Model file for the job. Use its own axes, mm. A direction names the side the tool comes from. Coordinates: 2 decimals unless noted, no trailing zeros. Order: outer loops, then holes, each group sorted by start corner. A loop starts at its lowest first (then second) coordinate and runs counter-clockwise, first axis right, second up. Notation, with made-up numbers: (5.5, 3) -> (30.5, 3) arc R27 cw to (30.5, 27) -> close; hole circle Ø1 at (87.5, 15). An arc over 180 degrees is marked (long way). Return JSON: item names as keys, results as strings. Group by question number.
1) Cut at B-B (z = 5). Write the cut outline in (x, y).
2) Flat gauge pins, fed straight in: pin 1 (5.5 mm diameter, centred on x = -1, y = 4, fed in from +Z); pin 2 (6 mm diameter, centred on x = -8, y = 9.5, fed in from +Z); pin 3 (5.5 mm diameter, centred on x = 14, z = 15, fed in from +Y); pin 4 (2 mm diameter, centred on x = -16, y = 5.5, fed in from +Z). Where does each tip first touch, or does it go through?
3) Cut at A-A (y = 5). Write the cut outline in (x, z).
4) Probe line 1 (Z direction, x = -14, y = 3.5); line 2 (Z direction, x = -12, y = 13.75); line 3 (X direction, y = 3.25, z = 57.5). List the from-to ranges inside material, lowest first.
5) Which spindle directions (+Z, -Z, +X, -X, +Y, -Y) get a long thin tool onto all of the face, cutting with end or side? Do faces 4 (the flat face through (0, 10, 11)), 5 (the cylindrical face through (10.925, 14.014, 126.686)), 6 (the flat face through (0.2, 9.3, 20)). Say none if no direction does.
6) Pull direction X, two halves, no side cores. Call faces 1 (the flat face through (-0.2, 9.3, 0)), 2 (the flat face through (-15.5, 6, 71)), 3 (the flat face through (-17.5, 8, 66)): +X half, -X half, draft (parallel to the pull), parting line (faces both ways), or undercut.
7) Cut at C-C (z = 76). Write the cut outline in (x, y).
8) Cut at D-D (x = -0.5). Write the cut outline in (y, z).
Autodesk Fusion 360 part; units mm, degrees
sketch "スケッチ1" plane through (0, 0, 0) normal (0, 0, 1) x (1, 0, 0)
  line L0 (-17.5, 15) -> (17.5, 15)
  line L1 (17.5, 15) -> (17.5, 0)
  line L2 (17.5, 0) -> (-17.5, 0)
  line L3 (-17.5, 0) -> (-17.5, 15)
  dimension "d1" = 35
  dimension "d2" = 15
extrude "押し出し1" add sketch "スケッチ1" along normal blind 120
sketch "スケッチ2" plane through (0, 0, 0) normal (0, 0, -1) x (1, 0, 0)
  line L0 (17.5, 0) -> (-17.5, 0)
  line L1 (-17.5, 0) -> (-17.5, -15)
  line L2 (-17.5, -15) -> (17.5, -15)
  line L3 (17.5, -15) -> (17.5, 0)
  circle A0 centre (0, 0) radius 9
  dimension "d5" = 18
extrude "押し出し2" cut sketch "スケッチ2" against normal blind 20 contours L0 A0 picked at (1.5, -2.5981)
sketch "スケッチ3" plane through (0, 0, 120) normal (0, 0, 1) x (-1, 0, 0)
  line L0 (17.5, 0) -> (-17.5, 0)
  line L1 (-17.5, 0) -> (-17.5, -15)
  line L2 (-17.5, -15) -> (17.5, -15)
  line L3 (17.5, -15) -> (17.5, 0)
  line L4 (15.5, -13) -> (-15.5, -13)
  line L5 (-15.5, -13) -> (-15.5, 0)
  line L6 (-15.5, 0) -> (15.5, 0)
  line L7 (15.5, 0) -> (15.5, -13)
  dimension "d8" = 2
  dimension "d9" = 31
extrude "押し出し3" cut sketch "スケッチ3" against normal blind 100 contours L0 L4 L5 L6 L7
ref_plane "作業平面1" through (0, 7.5, 9) normal (0, 0, -1) x (-1, 0, 0)
sketch "スケッチ4" plane through (0, 6, 9) normal (0, 0, -1) x (1, 0, 0)
  line L0 (-17.5, 6) -> (17.5, 6)
  line L1 (17.5, 6) -> (17.5, -5)
  line L2 (17.5, -5) -> (-17.5, -5)
  line L3 (-17.5, -5) -> (-17.5, 6)
  line L4 (-17.5, 6) -> (-17.5, -9)
  line L5 (17.5, -9) -> (17.5, 6)
  line L6 (17.5, 6) -> (9, 6)
  dimension "d13" = 11
extrude "押し出し4" cut sketch "スケッチ4" against normal blind 2
sketch "スケッチ5" plane through (0, 15, 0) normal (0, 1, 0) x (-1, 0, 0)
  line L0 (-17.5, 0) -> (17.5, 0)
  line L1 (17.5, 0) -> (17.5, 120)
  line L2 (17.5, 120) -> (-17.5, 120)
  line L3 (-17.5, 120) -> (-17.5, 0)
  line L4 (-17.5, 130) -> (17.5, 130)
  line L5 (17.5, 130) -> (17.5, 120)
  line L6 (17.5, 120) -> (-17.5, 120)
  line L7 (-17.5, 120) -> (-17.5, 130)
  line L8 (-17.5, 125) -> (17.5, 125) construction
  circle A0 centre (12, 125) radius 2
  circle A1 centre (-12, 125) radius 2
  dimension "d16" = 4
  dimension "d17" = 4
  dimension "d18" = 24
  dimension "d19" = 10
  dimension "d20" = 5.5
extrude "押し出し5" add sketch "スケッチ5" against normal blind 2 contours L2 L4 L5 L6 L7
sketch "スケッチ7" plane through (0, 0, 0) normal (0, -1, 0) x (1, 0, 0)
  line L0 (-17.5, 11) -> (-9, 11)
  line L1 (-9, 11) -> (-9, 20)
  line L2 (-9, 20) -> (-15.5, 20)
  line L3 (-15.5, 20) -> (-15.5, 120)
  line L4 (-15.5, 120) -> (-17.5, 120)
  line L5 (-17.5, 120) -> (-17.5, 11)
  line L6 (-17.5, 11) -> (-16, 11)
  line L7 (-16, 11) -> (-16, 9)
  line L8 (-16, 9) -> (-17.5, 9)
  line L9 (-17.5, 9) -> (-17.5, 11)
  line L10 (-9, 9) -> (-17.5, 9)
  line L11 (17.5, 11) -> (16, 11)
  line L12 (16, 11) -> (16, 9)
  line L13 (16, 9) -> (17.5, 9)
  line L14 (17.5, 9) -> (17.5, 11)
  line L15 (17.5, 9) -> (9, 9)
  point P0 (17.5, 11)
  dimension "d26" = 32
  dimension "d27" = 1.5
extrude "押し出し7" add sketch "スケッチ7" against normal blind 11 contours L0 L6 L7 L8 L9 L10 | L11 L12 L13 L14 L15
sketch "スケッチ8" plane through (0, 0, 0) normal (0, -1, 0) x (1, 0, 0)
  line L0 (-16, 11) -> (-9, 11)
  line L1 (-9, 11) -> (-9, 20)
  line L2 (-9, 20) -> (-15.5, 20)
  line L3 (-15.5, 20) -> (-15.5, 120)
  line L4 (-15.5, 120) -> (-17.5, 120)
  line L5 (-17.5, 120) -> (-17.5, 0)
  line L6 (-17.5, 0) -> (-9, 0)
  line L7 (-9, 0) -> (-9, 9)
  line L8 (-9, 9) -> (-16, 9)
  line L9 (-16, 9) -> (-16, 11)
  circle A0 centre (-14, 15) radius 1.75
  line L10 (18.5, 15) -> (-17.5, 15) construction
  line L11 (17.541, 5) -> (-17.5, 5) construction
  line L12 (15.5, 20) -> (9, 20) construction
  circle A1 centre (14, 15) radius 1.75
  circle A2 centre (14, 5) radius 1.75
  circle A3 centre (-14, 5) radius 1.75
  line L13 (17.5, 0) -> (17.5, 120)
  dimension "d30" = 5
  dimension "d31" = 10
  dimension "d32" = 3.5
  dimension "d33" = 3.5
  dimension "d34" = 3.5
  dimension "d35" = 3.5
  dimension "d36" = 3.5
  dimension "d37" = 3.5
  dimension "d38" = 3.5
  dimension "d39" = 3.5
extrude "押し出し8" cut sketch "スケッチ8" against normal blind 15 contours A0 | A1 | A2 | A3
Answers below:
{
 "1": {"outline": "(-17.5, 0) -> (-15.75, 0) -> (-15.75, 15) -> (-17.5, 15) -> close; (-12.25, 0) -> (-9, 0) arc R9 cw to (9, 0) -> (12.25, 0) -> (12.25, 15) -> (-12.25, 15) -> close; (15.75, 0) -> (17.5, 0) -> (17.5, 15) -> (15.75, 15) -> close"},
 "2": {"pin 1": "passes through", "pin 2": "stops at z = 20", "pin 3": "stops at y = 15", "pin 4": "stops at z = 120"},
 "3": {"outline": "(-17.5, 0) -> (-7.48, 0) -> (-7.48, 9) -> (-16, 9) -> (-16, 11) -> (-7.48, 11) -> (-7.48, 20) -> (-15.5, 20) -> (-15.5, 120) -> (-17.5, 120) -> close; (7.48, 0) -> (17.5, 0) -> (17.5, 120) -> (15.5, 120) -> (15.5, 20) -> (7.48, 20) -> (7.48, 11) -> (16, 11) -> (16, 9) -> (7.48, 9) -> close; hole circle Ø3.5 at (-14, 5); hole circle Ø3.5 at (-14, 15); hole circle Ø3.5 at (14, 5); hole circle Ø3.5 at (14, 15)"},
 "4": {"line 1": "z = 0 to 3.25, 6.75 to 9, 11 to 13.25, 16.75 to 20", "line 2": "z = 0 to 123, 127 to 130", "line 3": "x = -17.5 to -15.5, 15.5 to 17.5"},
 "5": {"face 4": "-Y", "face 5": "+Y, -Y", "face 6": "+Z, -Y"},
 "6": {"face 1": "draft", "face 2": "undercut", "face 3": "-X half"},
 "7": {"outline": "(-17.5, 0) -> (-15.5, 0) -> (-15.5, 13) -> (15.5, 13) -> (15.5, 0) -> (17.5, 0) -> (17.5, 15) -> (-17.5, 15) -> close"},
 "8": {"outline": "(8.99, 0) -> (15, 0) -> (15, 130) -> (13, 130) -> (13, 20) -> (8.99, 20) -> (8.99, 11) -> (11, 11) -> (11, 9) -> (8.99, 9) -> close"}
}
